Work out the finished part from the listing and answer in its coordinate system (mm). A direction names the side the tool comes from. Round coordinates to 2 decimals unless told otherwise and drop trailing zeros. Order: outer loops, then holes, each group sorted by start corner. A loop starts at its lowest first (then second) coordinate and runs counter-clockwise, first axis right, second up. Notation, with made-up numbers: M 80.25,-30 L 99.25,-30 A12 cw 99.25,-21 Z; hole C -40,42 d9. An arc over 180 degrees is marked long. Return JSON: item names as keys, results as strings.
from build123d import *

# Parameters (mm, degrees)
BOSS_EXTRUDE1_DEPTH      = 92
SKETCH2_4_W              = 5
SKETCH2_4_H              = 29
SKETCH2_4_W_2            = 58
SKETCH2_4_H_2            = 11
BOSS_EXTRUDE2_DEPTH      = 5
SKETCH2_6_W              = 5
SKETCH2_6_H              = 29
BOSS_EXTRUDE3_DEPTH      = 53
BOSS_EXTRUDE4_DEPTH      = 5
SKETCH6_W                = 3.75
SKETCH6_H                = 5
CUT_EXTRUDE1_DEPTH       = 29
BOSS_EXTRUDE5_DEPTH      = 3
BOSS_EXTRUDE6_DEPTH      = 13
SKETCH9_W                = 58
SKETCH9_H                = 11
BOSS_EXTRUDE7_DEPTH      = 5
SKETCH13_W               = 3
SKETCH13_H               = 44
BOSS_EXTRUDE9_DEPTH      = 10
FILLET1_R                = 2
CUT_EXTRUDE2_START       = -97
CUT_EXTRUDE2_OUTLINE_W   = 7.5
CUT_EXTRUDE2_OUTLINE_H   = 11
CUT_EXTRUDE2_OUTLINE_W_2 = 21
CUT_EXTRUDE2_DEPTH       = 97
SKETCH11_W               = 6
SKETCH11_H               = 5
BOSS_EXTRUDE8_DEPTH      = 35
FILLET2_R                = 2


# Read off the part's stored shape, not the designer's step: Cut-Extrude2
with BuildPart() as part:
    # Sketch2 → Boss-Extrude1 (new body)
    with BuildSketch(Plane.XY):
        Polygon((0, 16), (-5, 16), (-5, 5), (-63, 5), (-63, 16), (-74, 16), (-74, 5), (-100, 5), (-100, 0), (0, 0), align=None)
    extrude(amount=BOSS_EXTRUDE1_DEPTH)

    # Sketch2<4> → Boss-Extrude2 (add)
    with BuildSketch(Plane.XY):
        Polygon((-74, 0), (-74, 5), (-95, 5), (-100, 5), (-100, 0), align=None)
        with Locations((-97.5, 19.5)):
            Rectangle(SKETCH2_4_W, SKETCH2_4_H)
        Polygon((-74, 5), (-74, 16), (-74, 34), (-95, 34), (-95, 5), align=None)
        with Locations((-34, 10.5)):
            Rectangle(SKETCH2_4_W_2, SKETCH2_4_H_2)
    extrude(amount=BOSS_EXTRUDE2_DEPTH)

    # Sketch2<6> → Boss-Extrude3 (add)
    with BuildSketch(Plane.XY):
        Polygon((-74, 0), (-74, 5), (-95, 5), (-100, 5), (-100, 0), align=None)
        with Locations((-97.5, 19.5)):
            Rectangle(SKETCH2_6_W, SKETCH2_6_H)
    extrude(amount=BOSS_EXTRUDE3_DEPTH)

    # Sketch3 → Boss-Extrude4 (add)
    with BuildSketch(Plane.XY.offset(53)):
        Polygon((-95, 34), (-95, 5), (-74, 5), (-74, 16), (-74, 34), align=None)
    extrude(amount=-BOSS_EXTRUDE4_DEPTH)

    # Sketch6 → Cut-Extrude1 (cut)
    with BuildSketch(Plane(origin=(0, 34, 0), x_dir=(1, 0, 0), z_dir=(0, 1, 0))):
        with Locations((-82.625, -2.5)):
            Rectangle(SKETCH6_W, SKETCH6_H)
        with Locations((-86.375, -2.5)):
            Rectangle(SKETCH6_W, SKETCH6_H)
    extrude(amount=-CUT_EXTRUDE1_DEPTH, mode=Mode.SUBTRACT)

    # Sketch7 → Boss-Extrude5 (add)
    with BuildSketch(Plane(origin=(0, 0, 0), x_dir=(1, 0, 0), z_dir=(0, 1, 0))):
        with BuildLine():
            ThreePointArc((-16, 18), (-21.272077939, 5.272077939), (-34, 0))
            Line((-34, 0), (-16, 0))
            Line((-16, 0), (-16, 18))
        make_face()
        with BuildLine():
            Line((-52, 0), (-34, 0))
            ThreePointArc((-34, 0), (-46.727922061, 5.272077939), (-52, 18))
            Line((-52, 18), (-52, 0))
        make_face()
        with BuildLine():
            ThreePointArc((-52, 18), (-46.727922061, 5.272077939), (-34, 0))
            Line((-34, 0), (-34, 2.5))
            ThreePointArc((-34, 2.5), (-49.5, 18), (-34, 33.5))
            Line((-34, 33.5), (-34, 36))
            ThreePointArc((-34, 36), (-46.727922061, 30.727922061), (-52, 18))
        make_face()
        with BuildLine():
            Line((-34, 2.5), (-34, 0))
            ThreePointArc((-34, 0), (-21.272077939, 5.272077939), (-16, 18))
            ThreePointArc((-16, 18), (-21.272077939, 30.727922061), (-34, 36))
            Line((-34, 36), (-34, 33.5))
            ThreePointArc((-34, 33.5), (-23.039844892, 28.960155108), (-18.5, 18))
            ThreePointArc((-18.5, 18), (-23.039844892, 7.039844892), (-34, 2.5))
        make_face()
        with BuildLine():
            ThreePointArc((-34, 33.5), (-49.5, 18), (-34, 2.5))
            Line((-34, 2.5), (-34, 33.5))
        make_face()
        with BuildLine():
            Line((-34, 33.5), (-34, 2.5))
            ThreePointArc((-34, 2.5), (-23.039844892, 7.039844892), (-18.5, 18))
            ThreePointArc((-18.5, 18), (-23.039844892, 28.960155108), (-34, 33.5))
        make_face()
    extrude(amount=BOSS_EXTRUDE5_DEPTH)

    # Sketch7<3> → Boss-Extrude6 (add)
    with BuildSketch(Plane(origin=(0, 0, 0), x_dir=(1, 0, 0), z_dir=(0, 1, 0))):
        with BuildLine():
            Line((-52, 0), (-34, 0))
            ThreePointArc((-34, 0), (-46.727922061, 5.272077939), (-52, 18))
            Line((-52, 18), (-52, 0))
        make_face()
        with BuildLine():
            ThreePointArc((-52, 18), (-46.727922061, 5.272077939), (-34, 0))
            Line((-34, 0), (-34, 2.5))
            ThreePointArc((-34, 2.5), (-49.5, 18), (-34, 33.5))
            Line((-34, 33.5), (-34, 36))
            ThreePointArc((-34, 36), (-46.727922061, 30.727922061), (-52, 18))
        make_face()
        with BuildLine():
            Line((-34, 2.5), (-34, 0))
            ThreePointArc((-34, 0), (-21.272077939, 5.272077939), (-16, 18))
            ThreePointArc((-16, 18), (-21.272077939, 30.727922061), (-34, 36))
            Line((-34, 36), (-34, 33.5))
            ThreePointArc((-34, 33.5), (-23.039844892, 28.960155108), (-18.5, 18))
            ThreePointArc((-18.5, 18), (-23.039844892, 7.039844892), (-34, 2.5))
        make_face()
        with BuildLine():
            ThreePointArc((-16, 18), (-21.272077939, 5.272077939), (-34, 0))
            Line((-34, 0), (-16, 0))
            Line((-16, 0), (-16, 18))
        make_face()
    extrude(amount=BOSS_EXTRUDE6_DEPTH)

    # Sketch9 → Boss-Extrude7 (add)
    with BuildSketch(Plane.XY.offset(92)):
        with Locations((-34, 10.5)):
            Rectangle(SKETCH9_W, SKETCH9_H)
        Polygon((-63, 16), (-74, 16), (-74, 5), (-100, 5), (-100, 0), (0, 0), (0, 16), (-5, 16), (-5, 5), (-63, 5), align=None)
    extrude(amount=BOSS_EXTRUDE7_DEPTH)

    # Sketch13 → Boss-Extrude9 (add)
    with BuildSketch(Plane(origin=(0, 5, 0), x_dir=(1, 0, 0), z_dir=(0, 1, 0))):
        with Locations((-92, -75)):
            Rectangle(SKETCH13_W, SKETCH13_H)
    extrude(amount=BOSS_EXTRUDE9_DEPTH)

    # Fillet1
    fillet1_edges = [part.edges().sort_by_distance(p)[0] for p in [
        (-100, 19.5, 53),
        (0, 8, 0),
        (-80.75, 34, 2.5),
        (-88.25, 34, 2.5),
        (-16, 6.5, 0),
        (-52, 6.5, 0),
        (-34, 13, -2.5),
        (-74, 10.5, 97),
        (-100, 2.5, 97),
        (0, 8, 97),
        (-100, 17, 0),
    ]]
    fillet(fillet1_edges, radius=FILLET1_R)

    # Cut-Extrude2 outline → Cut-Extrude2 (cut)
    with BuildSketch(Plane.XY.offset(97).offset(CUT_EXTRUDE2_START)):
        with Locations((-13.75, 10.5)):
            Rectangle(CUT_EXTRUDE2_OUTLINE_W, CUT_EXTRUDE2_OUTLINE_H)
        with Locations((-34, 10.5)):
            Rectangle(CUT_EXTRUDE2_OUTLINE_W_2, CUT_EXTRUDE2_OUTLINE_H)
        with Locations((-54.25, 10.5)):
            Rectangle(CUT_EXTRUDE2_OUTLINE_W, CUT_EXTRUDE2_OUTLINE_H)
    extrude(amount=CUT_EXTRUDE2_DEPTH, mode=Mode.SUBTRACT)

    # Sketch11 → Boss-Extrude8 (add)
    with BuildSketch(Plane(origin=(0, 16, 0), x_dir=(1, 0, 0), z_dir=(0, 1, 0))):
        with Locations((-20.5, -2.5)):
            Rectangle(SKETCH11_W, SKETCH11_H)
        with Locations((-47.5, -2.5)):
            Rectangle(SKETCH11_W, SKETCH11_H)
    extrude(amount=BOSS_EXTRUDE8_DEPTH)

    # Fillet2
    fillet2_edges = [part.edges().sort_by_distance(p)[0] for p in [
        (-90.5, 10, 97),
        (-10, 10.5, 97),
        (-17.5, 10.5, 97),
        (-10, 10.5, 0),
        (-17.5, 5, 2.5),
        (-17.5, 9, 0),
        (-58, 10.5, 0),
        (-58, 10.5, 97),
        (-50.5, 9, 0),
        (-50.5, 5, 2.5),
        (-44.5, 32, 0),
        (-23.5, 10.5, 97),
        (-23.5, 5, 2.5),
        (-44.5, 5, 2.5),
        (-44.5, 10.5, 97),
        (-23.5, 32, 0),
        (-20.5, 51, 0),
        (-20.5, 51, 5),
        (-47.5, 51, 0),
        (-47.5, 51, 5),
    ]]
    fillet(fillet2_edges, radius=FILLET2_R)


solid = part.part
Item 1: Consider line 1 along X through (y, z) = (5.5, 77); line 2 along Y through (x, z) = (-53.5, 32); line 3 along X through (y, z) = (17.5, 37.5). Determine where each line is inside the solid, lowest interval first. Write a range as [from, to].
Output:
{"line 1": "x = [-93.5, -90.5], [-74, -63], [-5, 0]", "line 2": "y = [0, 5]", "line 3": "x = [-100, -95]"}
Item 2: Find section B-B (z = 46). Determine the outline of the cut face in (x, y).
Output:
{"outline": "M -100,0 L 0,0 L 0,16 L -5,16 L -5,5 L -63,5 L -63,16 L -74,16 L -74,5 L -95,5 L -95,34 L -100,34 Z"}
Item 3: Find section C-C (x = -68). Determine the outline of the cut face in (y, z).
Output:
{"outline": "M 0,0 L 16,0 L 16,97 L 0,97 Z"}
Item 4: Find section A-A (y = 47). Determine the outline of the cut face in (x, z).
Output:
{"outline": "M -50.5,0 L -46.5,0 A2 ccw -44.5,2 L -44.5,5 L -50.5,5 Z; M -23.5,2 A2 ccw -21.5,0 L -17.5,0 L -17.5,5 L -23.5,5 Z"}
Item 5: Which of the six approach directions +Z, -Z, +X, -X, +Y, -Y give full straight-line access (tool end or side, diameter ignored) to faces 4 (the flat face through (-93.5, 10, 75)), 5 (the flat face through (-20, 16, 94)), 6 (the flat face through (-8, 11, 5))?
Output:
{"face 4": "+Z, -X, +Y", "face 5": "+Z, +X, -X, +Y", "face 6": "+Y"}
Item 6: Each of these flat-tipped pins is pushed along its axis until it touches: pin 1 (2.5 mm diameter, centred on x = -8.5, y = 10, fed in from -Z); pin 2 (2.5 mm diameter, centred on x = -76, z = 1.5, fed in from +Y); pin 3 (2.5 mm diameter, centred on y = 35.5, z = 2.5, fed in from +X). Where does it stop, or does it pass through?
Output:
{"pin 1": "stops at z = 0", "pin 2": "stops at y = 34", "pin 3": "stops at x = -17.5"}
Item 7: The mould has two halves that part along X. Classify faces 1 (the flat face through (-97, 5, 74)), 2 (the flat face through (-23.5, 29, 4)), 3 (the flat face through (-100, 17, 27)): pulls with the +X half, pulls with the -X half, needs draft (parallel to the pull), parting line crosses it, or undercut.
Output:
{"face 1": "needs draft", "face 2": "undercut", "face 3": "pulls with the -X half"}
